Verification items for the finished model (mm, model axes). Face numbers are marked on the shaded views. A direction names the side the tool comes from. Round coordinates to 2 decimals unless told otherwise and drop trailing zeros. Write each loop counter-clockwise with the first axis right and the second up, starting at its lowest first coordinate (ties: lowest second). Pieces come first, ordered by that corner, then holes. Notation, with made-up numbers: (8, 81) - (43, 81) arc R33 cw to (43, 120) - close; hole circle Ø3 at (-28, 77.5). An arc over 180 degrees is marked (long way). Write each question's results on one line, items separated by ' | '.
```python
from build123d import *

# Parameters (mm, degrees)
F0_W     = 9
F0_H     = 11
F1_DEPTH = 3.45
F3_DEPTH = 11
F4_R     = 3.2
F5_DEPTH = 9
F6_R     = 1
F7_DEPTH = 8
F8_R     = 0.25


with BuildPart() as f1:
    # F0 (on Front) → F1 (new body)
    with BuildSketch(Plane.XZ):
        with Locations((0, -1)):
            Rectangle(F0_W, F0_H)
    extrude(amount=-F1_DEPTH)

    # F2 (on face) → F3 (join)
    with BuildSketch(Plane(origin=(0, 3.45, 0), x_dir=(-1, 0, 0), z_dir=(0, 1, 0))):
        with BuildLine():
            ThreePointArc((4, 0), (0, 4), (-4, 0))
            Line((-4, 0), (-4.5, 0))
            Line((-4.5, 0), (-4.5, -6.5))
            Line((-4.5, -6.5), (4.5, -6.5))
            Line((4.5, -6.5), (4.5, 0))
            Line((4.5, 0), (4, 0))
        make_face()
    extrude(amount=F3_DEPTH)

    # F4 (on face) → F5 (cut)
    with BuildSketch(Plane.XZ):
        Circle(F4_R)
    extrude(amount=-F5_DEPTH, mode=Mode.SUBTRACT)

    # F6 (on face) → F7 (join)
    with BuildSketch(Plane.XZ.offset(-9)):
        Circle(F6_R)
    extrude(amount=F7_DEPTH)

    # F8
    f8_edges = [f1.edges().sort_by_distance(p)[0] for p in [
        (-1, 1, 0),
    ]]
    fillet(f8_edges, radius=F8_R)


solid = f1.part
```
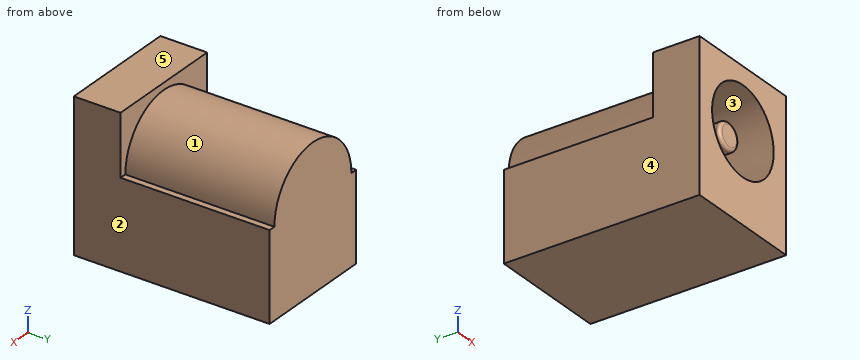
(1) Mould release check, pull along X, two halves, no side actions. Record for the marked faces 3, 4 and 5: released by +X, released by -X, zero draft, split by the parting line, or undercut.
Answer:
face 3: undercut | face 4: released by -X | face 5: zero draft
(2) Go/stop test with flat-tipped pins: pin 1 Ø0.6 at (x, y) = (-4, 9.5) entering from +Z; pin 2 Ø0.8 at (x, z) = (0, -0.5) entering from -Y; pin 3 Ø3 at (x, y) = (1, 11) entering from +Z. Record where each tip stops, or that it passes through.
Answer:
pin 1: z = 1.52 | pin 2: y = 1 | pin 3: z = 4
(3) Section check A-A (x = 0). Record the cut outline in (y, z).
Answer:
outline: (0, -6.5) - (14.45, -6.5) - (14.45, 4) - (3.45, 4) - (3.45, 4.5) - (0, 4.5) - (0, 3.2) - (9, 3.2) - (9, 1) - (1.25, 1) arc R0.25 ccw to (1, 0.75) - (1, -0.75) arc R0.25 ccw to (1.25, -1) - (9, -1) - (9, -3.2) - (0, -3.2) - close
(4) Section check B-B (y = 11). Record the cut outline in (x, z), plus the area to 3 significant figures.
Answer:
outline: (-4.5, -6.5) - (4.5, -6.5) - (4.5, 0) - (4, 0) arc R4 ccw to (-4, 0) - (-4.5, 0) - close | area: 83.6 mm2
(5) Thickness scan on L1, parallel to Z at x = 0, y = 4.25; L2, parallel to Z at x = 0, y = 2.75; L3, parallel to Y at x = 1.5, z = -0.5. Record the ranges inside material, lowest first.
Answer:
L1: -6.5 to -3.2, -1 to 1, 3.2 to 4 | L2: -6.5 to -3.2, -1 to 1, 3.2 to 4.5 | L3: 9 to 14.45
(6) Section check D-D (x = -1.25). Record the cut outline in (y, z).
Answer:
outline: (0, -6.5) - (14.45, -6.5) - (14.45, 3.8) - (3.45, 3.8) - (3.45, 4.5) - (0, 4.5) - (0, 2.95) - (9, 2.95) - (9, -2.95) - (0, -2.95) - close
(7) Set-up check for the marked faces 1 and 2: record each of +Z, -Z, +X, -X, +Y, -Y from which the full face is reachable in a straight line by a thin tool's end or side.
Answer:
face 1: +Z, +Y | face 2: +Z, -Z, +X, +Y, -Y
(8) Section check C-C (z = 3). Record the cut outline in (x, y), plus the area to 3 significant figures.
Answer:
outline: (-4.5, 0) - (-1.11, 0) - (-1.11, 9) - (1.11, 9) - (1.11, 0) - (4.5, 0) - (4.5, 3.45) - (2.65, 3.45) - (2.65, 14.45) - (-2.65, 14.45) - (-2.65, 3.45) - (-4.5, 3.45) - close | area: 69.2 mm2
